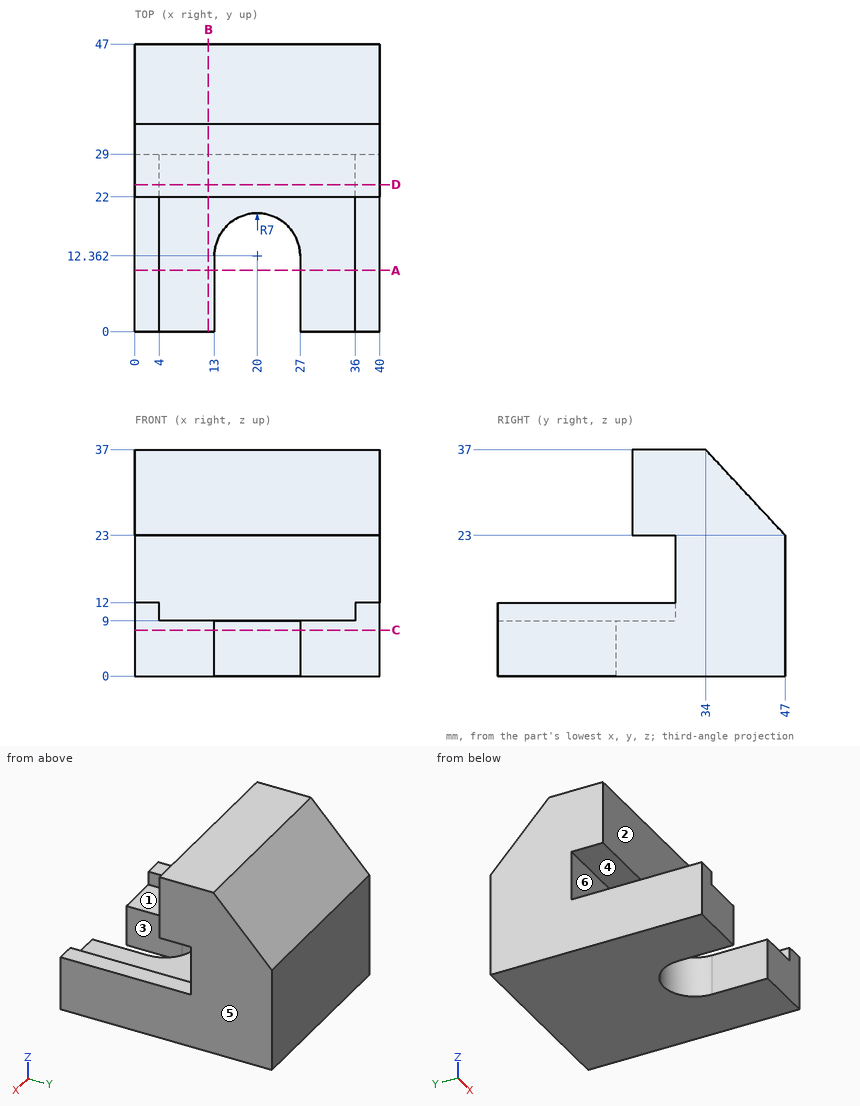
Here's the drawing with two shaded views (mm, measured from the low corner). I have some questions. A direction names the side the tool comes from. Give positions to 0.01 mm unless a question says otherwise; leave off trailing zeros. Order: outer loops, then holes, each group sorted by start corner. A loop starts at its lowest first (then second) coordinate and runs counter-clockwise, first axis right, second up. Notation, with made-up numbers: (68, 5) - (73, 5) arc R32 ccw to (73, 31) - close; hole circle Ø11 at (70.25, 47.5). An arc over 180 degrees is marked (long way). Use a Markdown table: item, result. Add a question column.
Q1. On a 3-axis mill with a long thin cutter (end or side, diameter ignored), from which of +Z, -Z, +X, -X, +Y, -Y can I reach the whole of each face in a straight line? I mean the marked faces 1, 2 and 3. Say none if no direction works.
Q2. If we section it at C-C on z = 7.5: Write out the boundary of the cut face in (x, y), plus the area to 3 significant figures.
Q3. If we section it at A-A on y = 10: Write out the boundary of the cut face in (x, z).
Q4. If we section it at B-B on x = 12: Write out the boundary of the cut face in (y, z).
Q5. If we mould it in two halves opening along X, with no side actions, what happens to the marked faces 4, 5 and 6? For each: released by +X, released by -X, zero draft, split by the parting line, or undercut.
Q6. Please list where these lines run through material, in increasing order: line 1 along Z through (x, y) = (29.5, 16); line 2 along Y through (x, z) = (33, 10); line 3 along X through (y, z) = (2.5, 10.5).
Q7. If we section it at D-D on y = 24: Write out the boundary of the cut face in (x, z).
Q8. I'm going to push flat-ended pins straight in: pin 1 (2 mm diameter, centred on x = 1.5, y = 16.5, fed in from +Z); pin 2 (7 mm diameter, centred on x = 15, z = 16.5, fed in from -Y); pin 3 (6 mm diameter, centred on x = 7.5, y = 41, fed in from +Z). Where does each tip first touch, or does it pass through?
Answers follow:
| question | item | result |
|---|---|---|
| 1 | face 1 | -Y |
| 1 | face 2 | +Z, +X, -X, -Y |
| 1 | face 3 | +Z, -Z, -Y |
| 2 | outline | (0, 0) - (13, 0) - (13, 12.36) arc R7 cw to (27, 12.36) - (27, 0) - (40, 0) - (40, 47) - (0, 47) - close |
| 2 | area | 1,630 mm^2 |
| 3 | outline | (0, 0) - (13, 0) - (13, 9) - (4, 9) - (4, 12) - (0, 12) - close; (27, 0) - (40, 0) - (40, 12) - (36, 12) - (36, 9) - (27, 9) - close |
| 4 | outline | (0, 0) - (47, 0) - (47, 23) - (34, 37) - (22, 37) - (22, 23) - (29, 23) - (29, 9) - (0, 9) - close |
| 5 | face 4 | zero draft |
| 5 | face 5 | released by +X |
| 5 | face 6 | undercut |
| 6 | line 1 | z = 0 to 9 |
| 6 | line 2 | y = 29 to 47 |
| 6 | line 3 | x = 0 to 4, 36 to 40 |
| 7 | outline | (0, 0) - (40, 0) - (40, 12) - (36, 12) - (36, 9) - (4, 9) - (4, 12) - (0, 12) - close; (0, 23) - (40, 23) - (40, 37) - (0, 37) - close |
| 8 | pin 1 | stops at z = 12 |
| 8 | pin 2 | stops at y = 29 |
| 8 | pin 3 | stops at z = 32.69 |
